from build123d import *

# Parameters (mm, degrees)
F0_R     = 12.319
F1_DEPTH = 33.02
F3_R     = 6.35
F4_DEPTH = 25.4
F5_R     = 0.254
F7_DEPTH = 3.81


with BuildPart() as f1:
    # F0 (on Front) → F1 (new body)
    with BuildSketch(Plane.XZ):
        Circle(F0_R)
    extrude(amount=F1_DEPTH)

    # F3 (on face) → F4 (cut)
    with BuildSketch(Plane.XZ.offset(33.02)):
        Circle(F3_R)
    extrude(amount=-F4_DEPTH, mode=Mode.SUBTRACT)

    # F5
    f5_edges = [f1.edges().sort_by_distance(p)[0] for p in [
        (-12.319, -33.02, 0),
        (-12.319, 0, 0),
    ]]
    fillet(f5_edges, radius=F5_R)

    # F6 (on face) → F7 (cut)
    with BuildSketch(Plane.XZ.offset(33.02)):
        with BuildLine():
            ThreePointArc((-1.27, 6.2217039467), (0, 6.35), (1.27, 6.2217039467))
            Line((1.27, 6.2217039467), (1.27, 12.2533612123))
            ThreePointArc((1.27, 12.2533612123), (0, 12.319), (-1.27, 12.2533612123))
            Line((-1.27, 12.2533612123), (-1.27, 6.2217039467))
        make_face()
        with BuildLine():
            Line((-6.2217039467, 1.27), (-12.2533612123, 1.27))
            ThreePointArc((-12.2533612123, 1.27), (-12.319, 0), (-12.2533612123, -1.27))
            Line((-12.2533612123, -1.27), (-6.2217039467, -1.27))
            ThreePointArc((-6.2217039467, -1.27), (-6.35, 0), (-6.2217039467, 1.27))
        make_face()
        with BuildLine():
            Line((-1.27, -6.2217039467), (-1.27, -12.2533612123))
            ThreePointArc((-1.27, -12.2533612123), (0, -12.319), (1.27, -12.2533612123))
            Line((1.27, -12.2533612123), (1.27, -6.2217039467))
            ThreePointArc((1.27, -6.2217039467), (0, -6.35), (-1.27, -6.2217039467))
        make_face()
        with BuildLine():
            Line((6.2217039467, -1.27), (12.2533612123, -1.27))
            ThreePointArc((12.2533612123, -1.27), (12.319, 0), (12.2533612123, 1.27))
            Line((12.2533612123, 1.27), (6.2217039467, 1.27))
            ThreePointArc((6.2217039467, 1.27), (6.35, 0), (6.2217039467, -1.27))
        make_face()
    extrude(amount=-F7_DEPTH, mode=Mode.SUBTRACT)


solid = f1.part
Could you check a few things on this model? Use its own coordinates, in mm. A direction names the side the tool comes from. Give positions to 0.01 mm unless a question says otherwise; leave off trailing zeros. Order: outer loops, then holes, each group sorted by start corner. A loop starts at its lowest first (then second) coordinate and runs counter-clockwise, first axis right, second up.
1. We'd pull the mould along X, two halves only. Please class faces 1 (the flat face through (-1.27, -31, -9)), 2 (the flat face through (-9, -31, -1.27)), 3 (the cylindrical face through (11.75, -16.28, 3.7)): pulls with the +X half, pulls with the -X half, needs draft (parallel to the pull), parting line crosses it, or undercut.
2. I need wall thicknesses on L1, parallel to X at y = -17.5, z = 0; L2, parallel to Z at x = 1.25, y = -12.5. Which ranges of each line are inside material? Lowest first, please.
3. Suppose I cut it at A-A (z = 0). List the corners of the cut face in (x, y) for me (3 decimals), plus the area to 3 significant figures.
4. Suppose I cut it at C-C (y = -15.5). List the corners of the cut face in (x, z) for me.
5. For faces 4 (the flat face through (9, -29.21, 0)), 5 (the flat face through (1.27, -31, -9)), 6 (the flat face through (0, -7.62, 0)), which set-ups out of +Z, -Z, +X, -X, +Y, -Y let a thin tool reach every point of the face, with its end or its side?
6. Will these pins go through, and if not, where does the flat tip stop? P1, Ø4, axis at y = -32, z = -9.5, coming from the +X side; P2, Ø7.5, axis at x = 0, z = 0, coming from the -Y side; P3, Ø4, axis at x = -10.5, y = -31.5, coming from the -Z side.
7. Suppose I cut it at B-B (x = 0). List the corners of the cut face in (y, z) for me (3 decimals).
Solved:
1. face 1: undercut
1. face 2: needs draft
1. face 3: parting line crosses it
2. L1: x = -12.32 to -6.35, 6.35 to 12.32
2. L2: z = -12.26 to -6.23, 6.23 to 12.26
3. outline: (-12.319, -29.21) - (-6.35, -29.21) - (-6.35, -7.62) - (6.35, -7.62) - (6.35, -29.21) - (12.319, -29.21) - (12.319, -0.254) arc R0.254 ccw to (12.065, 0) - (-12.065, 0) arc R0.254 ccw to (-12.319, -0.254) - close
3. area: 445 mm2
4. outline: circle Ø24.64 at (0, 0); hole circle Ø12.7 at (0, 0)
5. face 4: +X, -X, -Y
5. face 5: +Z, -Z, -Y
5. face 6: -Y
6. P1: stops at x = 9.77
6. P2: stops at y = -7.62
6. P3: stops at z = -8.92
7. outline: (-29.21, -12.319) - (-0.254, -12.319) arc R0.254 ccw to (0, -12.065) - (0, 12.065) arc R0.254 ccw to (-0.254, 12.319) - (-29.21, 12.319) - (-29.21, 6.35) - (-7.62, 6.35) - (-7.62, -6.35) - (-29.21, -6.35) - close
